Autodesk Inventor part; units mm, degrees
ref_plane "YZ Plane" through (0, 0, 0) normal (1, 0, 0) x (0, 1, 0)
ref_plane "XZ Plane" through (0, 0, 0) normal (0, 1, 0) x (-1, 0, 0)
ref_plane "XY Plane" through (0, 0, 0) normal (0, 0, 1) x (1, 0, 0)
sketch "Sketch1" plane through (0, 0, 0) normal (0, 1, 0) x (-1, 0, 0)
  line L0 (0, 0) -> (-400, 0)
  line L1 (-400, 0) -> (-400, 300)
  line L2 (-400, 300) -> (0, 300)
  line L3 (0, 300) -> (0, 0)
  line L4 (0, 300) -> (-20, 300)
  line L5 (-400, 300) -> (-380, 300)
  line L6 (-380, 300) -> (-380, 700)
  line L7 (-380, 700) -> (-400, 700)
  line L8 (-400, 700) -> (-400, 300)
  point P0 (-380, 300)
  dimension "d0" = 400
  dimension "d1" = 300
  dimension "d9" = 400
  dimension "d10" = 20
extrude "Extrusion1" add sketch "Sketch1" along normal blind 2100
sketch "Sketch3" plane through (0, 0, 0) normal (0, 1, 0) x (-1, 0, 0)
  line L0 (0, 300) -> (-380, 300)
  line L1 (-380, 300) -> (-380, 700)
  line L2 (-380, 700) -> (-400, 700)
  line L3 (-400, 700) -> (-400, 0)
  line L4 (-400, 0) -> (0, 0)
  line L5 (0, 0) -> (0, 300)
  arc A0 (0, 300) -> (-380, 700) centre (-380, 319.5) ccw
  arc A1 (-50.0758, 300) -> (-380, 650) centre (-380, 319.5) ccw
  dimension "d11" = 50
extrude "Extrusion3" add sketch "Sketch3" along normal blind 10 contours L0 A1 L1 A0
mirror "Mirror1" about plane through (0, 0, 0) normal (-1, 0, 0) of "Extrusion1", "Extrusion3"
equation "\"d9\" = d0"
properties part number "Electrical box 4"
Geometry check sheet. Reference: the model listing, model coordinates, mm. A direction names the side the tool comes from. Round coordinates to 2 decimals unless told otherwise and drop trailing zeros. Order: outer loops, then holes, each group sorted by start corner. A loop starts at its lowest first (then second) coordinate and runs counter-clockwise, first axis right, second up. Notation, with made-up numbers: (-18, -5.75) - (5, -5.75) arc R28 cw to (5, 20.25) - close; hole circle Ø8 at (80, -34.5). An arc over 180 degrees is marked (long way). Use a Markdown table: item, result. Add a question column.
(1) Material ranges on line 1 along X through (y, z) = (603, 436.5); line 2 along Z through (x, y) = (-309, 188); line 3 along Y through (x, z) = (183.5, 605), recorded low to high. Write a range as [from, to].
(2) Depth check by flat-ended pin: pin 1 (3 mm diameter, centred on x = 261, y = 612.5, fed in from +Z). Enter the tip coordinate at first touch or a pass-through.
(3) Sectioned sample at A-A, the plane z = 553. Enter the section's corners in (x, y), and give its area (3 significant figures).
(4) Sectioned sample at C-C, the plane y = 1109. Enter the section's corners in (x, z), and give its area (3 significant figures).
(5) Sectioned sample at D-D, the plane z = 396. Enter the section's corners in (x, y).
(6) Tool access check on faces 4 (the cylindrical face through (-136.935, 4.93, 543.441)), 5 (the flat face through (6, 0, 277)). Record the directions out of +Z, -Z, +X, -X, +Y, -Y that give a thin tool (end or side, any length) a straight path to the whole face; none if there is none.
(7) Sectioned sample at B-B, the plane x = 179.5. Enter the section's corners in (y, z), and give its area (3 significant figures).
(8) Release check for a two-part mould opening along Z. For faces 1 (the flat face through (-6, 1035, 0)), 2 (the cylindrical face through (142.11, 4.93, 548.93)), 3 (the flat face through (58, 10, 516)) record: pulls with the +Z half, pulls with the -Z half, needs draft (parallel to the pull), parting line crosses it, or undercut.
Answers below:
| question | item | result |
|---|---|---|
| 1 | line 1 | [-400, -380], [380, 400] |
| 1 | line 2 | [0, 300] |
| 1 | line 3 | [0, 10] |
| 2 | pin 1 | z = 300 |
| 3 | outline | (-400, 0) - (-380, 0) - (-380, 2100) - (-400, 2100) - close; (-146.1, 0) - (-79.57, 0) - (-79.57, 10) - (-146.1, 10) - close; (79.57, 0) - (146.1, 0) - (146.1, 10) - (79.57, 10) - close; (380, 0) - (400, 0) - (400, 2100) - (380, 2100) - close |
| 3 | area | 85,300 mm² |
| 4 | outline | (-400, 0) - (400, 0) - (400, 700) - (380, 700) - (380, 300) - (-380, 300) - (-380, 700) - (-400, 700) - close |
| 4 | area | 256,000 mm² |
| 5 | outline | (-400, 0) - (-380, 0) - (-380, 2100) - (-400, 2100) - close; (-58.48, 0) - (-7.27, 0) - (-7.27, 10) - (-58.48, 10) - close; (7.27, 0) - (58.48, 0) - (58.48, 10) - (7.27, 10) - close; (380, 0) - (400, 0) - (400, 2100) - (380, 2100) - close |
| 6 | face 4 | +Y, -Y |
| 6 | face 5 | +Z, -Z, +X, -X, -Y |
| 7 | outline | (0, 0) - (2100, 0) - (2100, 300) - (0, 300) - close; (0, 582.24) - (10, 582.24) - (10, 642.89) - (0, 642.89) - close |
| 7 | area | 631,000 mm² |
| 8 | face 1 | pulls with the -Z half |
| 8 | face 2 | undercut |
| 8 | face 3 | needs draft |
